Autodesk Fusion 360 part; units mm, degrees
sketch "Sketch1" plane through (0, 0, 0) normal (0, 0, 1) x (1, 0, 0)
  arc A0 (39.26, -24.3675) -> (42.26, -21.3675) centre (39.26, -21.3675) ccw
  circle A1 centre (38.26, -0.0995) radius 1.525
  circle A2 centre (-38.26, -20.3675) radius 1.75
  circle A3 centre (-38.26, 20.3675) radius 1.75
  line L0 (42.26, 21.3675) -> (42.26, -21.3675)
  arc A4 (-42.26, -21.3675) -> (-39.26, -24.3675) centre (-39.26, -21.3675) ccw
  line L1 (39.26, -24.3675) -> (-39.26, -24.3675)
  line L2 (-42.26, -21.3675) -> (-42.26, 21.3675)
  arc A5 (-39.26, 24.3675) -> (-42.26, 21.3675) centre (-39.26, 21.3675) ccw
  arc A6 (42.26, 21.3675) -> (39.26, 24.3675) centre (39.26, 21.3675) ccw
  circle A7 centre (38.26, 20.3675) radius 1.75
  circle A8 centre (-38.26, -0.0995) radius 1.525
  circle A9 centre (38.26, -20.3675) radius 1.75
  arc A10 (16.525, -9.1875) -> (15.025, -7.6875) centre (15.025, -9.1875) ccw
  arc A11 (-35.575, -12.1875) -> (-34.075, -13.6875) centre (-34.075, -12.1875) ccw
  line L3 (4.025, -7.6875) -> (15.025, -7.6875)
  arc A12 (-15.025, -7.6875) -> (-16.525, -9.1875) centre (-15.025, -9.1875) ccw
  line L4 (-16.525, -12.1875) -> (-16.525, -9.1875)
  line L5 (23.075, -13.6875) -> (34.075, -13.6875)
  line L6 (-15.025, -13.6875) -> (-4.025, -13.6875)
  arc A13 (21.575, -12.1875) -> (23.075, -13.6875) centre (23.075, -12.1875) ccw
  line L7 (-34.075, -7.6875) -> (-23.075, -7.6875)
  arc A14 (34.075, -13.6875) -> (35.575, -12.1875) centre (34.075, -12.1875) ccw
  line L8 (-34.075, -13.6875) -> (-23.075, -13.6875)
  line L9 (2.525, -12.1875) -> (2.525, -9.1875)
  arc A15 (35.575, -9.1875) -> (34.075, -7.6875) centre (34.075, -9.1875) ccw
  arc A16 (-2.525, -9.1875) -> (-4.025, -7.6875) centre (-4.025, -9.1875) ccw
  arc A17 (4.025, -7.6875) -> (2.525, -9.1875) centre (4.025, -9.1875) ccw
  line L10 (-35.575, -12.1875) -> (-35.575, -9.1875)
  line L11 (16.525, -12.1875) -> (16.525, -9.1875)
  arc A18 (-4.025, -13.6875) -> (-2.525, -12.1875) centre (-4.025, -12.1875) ccw
  line L12 (23.075, -7.6875) -> (34.075, -7.6875)
  arc A19 (-23.075, -13.6875) -> (-21.575, -12.1875) centre (-23.075, -12.1875) ccw
  line L13 (21.575, -12.1875) -> (21.575, -9.1875)
  line L14 (-15.025, -7.6875) -> (-4.025, -7.6875)
  line L15 (35.575, -12.1875) -> (35.575, -9.1875)
  arc A20 (2.525, -12.1875) -> (4.025, -13.6875) centre (4.025, -12.1875) ccw
  arc A21 (-16.525, -12.1875) -> (-15.025, -13.6875) centre (-15.025, -12.1875) ccw
  arc A22 (-21.575, -9.1875) -> (-23.075, -7.6875) centre (-23.075, -9.1875) ccw
  line L16 (-21.575, -12.1875) -> (-21.575, -9.1875)
  line L17 (-2.525, -12.1875) -> (-2.525, -9.1875)
  arc A23 (15.025, -13.6875) -> (16.525, -12.1875) centre (15.025, -12.1875) ccw
  arc A24 (-34.075, -7.6875) -> (-35.575, -9.1875) centre (-34.075, -9.1875) ccw
  line L18 (4.025, -13.6875) -> (15.025, -13.6875)
  arc A25 (23.075, -7.6875) -> (21.575, -9.1875) centre (23.075, -9.1875) ccw
  line L19 (-18.69, 4.8975) -> (-18.69, 13.8975)
  arc A26 (-18.69, 13.8975) -> (-21.69, 16.8975) centre (-21.69, 13.8975) ccw
  line L20 (-21.69, 16.8975) -> (-34.69, 16.8975)
  arc A27 (-34.69, 16.8975) -> (-37.69, 13.8975) centre (-34.69, 13.8975) ccw
  line L21 (-37.69, 4.8975) -> (-37.69, 13.8975)
  arc A28 (-37.69, 4.8975) -> (-34.69, 1.8975) centre (-34.69, 4.8975) ccw
  line L22 (-21.69, 1.8975) -> (-34.69, 1.8975)
  arc A29 (-21.69, 1.8975) -> (-18.69, 4.8975) centre (-21.69, 4.8975) ccw
  line L23 (35, -3.4325) -> (15, -3.4325)
  line L24 (19.67, 23.0675) -> (15, 23.0675)
  line L25 (30.33, 23.0675) -> (35, 23.0675)
  line L26 (15, -3.4325) -> (15, 23.0675)
  line L27 (35, 23.0675) -> (35, -3.4325)
  line L28 (19.67, 23.0675) -> (19.67, 24.3675)
  line L29 (30.33, 23.0675) -> (30.33, 24.3675)
  line L30 (39.26, 24.3675) -> (30.33, 24.3675)
  line L31 (19.67, 24.3675) -> (-39.26, 24.3675)
  point P0 (-42.26, -24.3675)
  dimension "d1" = 3.5
  dimension "d2" = 3.05
  dimension "d3" = 3.05
  dimension "d4" = 20.268
  dimension "d5" = 3
  dimension "d6" = 3
  dimension "d7" = 3
  dimension "d8" = 3
  dimension "d11" = 3.5
  dimension "d12" = 1.4142
  dimension "d13" = 4
  dimension "d14" = 10.68
  dimension "d15" = 6
  dimension "d16" = 14
  dimension "d17" = 1.5
  dimension "d18" = 1.5
  dimension "d19" = 1.5
  dimension "d20" = 1.5
  dimension "d21" = 1.5
  dimension "d22" = 1.5
  dimension "d23" = 1.5
  dimension "d24" = 1.5
  dimension "d25" = 1.5
  dimension "d26" = 1.5
  dimension "d27" = 1.5
  dimension "d28" = 1.5
  dimension "d29" = 1.5
  dimension "d30" = 1.5
  dimension "d31" = 1.5
  dimension "d32" = 1.5
  dimension "d33" = 6
  dimension "d34" = 6
  dimension "d35" = 6
  dimension "d36" = 10.68
  dimension "d37" = 10.68
  dimension "d38" = 10.68
  dimension "d40" = 6.685
  dimension "d41" = 5.05
  dimension "d42" = 5.05
  dimension "d43" = 5.05
  dimension "d44" = 4
  dimension "d45" = 4
  dimension "d46" = 4
  dimension "d47" = 1.4142
  dimension "d48" = 4
  dimension "d49" = 1.4142
  dimension "d50" = 20.268
  dimension "d51" = 14
  dimension "d52" = 14
  dimension "d53" = 14
  dimension "d54" = 6.685
  dimension "d55" = 3
  dimension "d56" = 3
  dimension "d57" = 3
  dimension "d58" = 3
  dimension "d59" = 19
  dimension "d60" = 15
  dimension "d61" = 4.57
  dimension "d63" = 26.5
  dimension "d64" = 26.5
  dimension "d65" = 20
  dimension "d66" = 10.66
  dimension "d67" = 1.3
  dimension "d68" = 1.3
  dimension "d69" = 4.67
  dimension "d70" = 4.67
  dimension "d71" = 7.26
  dimension "d78" = 3.5
  dimension "d79" = 3.5
extrude "Extrude1" add sketch "Sketch1" along normal blind 3
extrude "Extrude2" add 1 faces at (0.0405, 9.7541, 3) along direction (0, 0, 1) blind 4
extrude "Extrude4" add 1 faces at (0.0405, 9.7541, 7) along direction (0, 0, 1) blind 1
Geometry: final body of the model. Coordinates: model frame, mm. A direction names the side the tool comes from. Give positions to 0.01 mm unless a question says otherwise; leave off trailing zeros. Order: outer loops, then holes, each group sorted by start corner. A loop starts at its lowest first (then second) coordinate and runs counter-clockwise, first axis right, second up. Notation, with made-up numbers: (31, 11) - (58, 11) arc R33 cw to (58, 43) - close; hole circle Ø9 at (36, 46). An arc over 180 degrees is marked (long way). Use CSV: the item, a comma, the result in double quotes.
1. Section query C-C (x = -13.5). Output: boundary loops of the cut face in (y, z), plus the area to 3 significant figures.
Answers below:
outline,"(-24.37, 0) - (-13.69, 0) - (-13.69, 8) - (-24.37, 8) - close; (-7.69, 0) - (24.37, 0) - (24.37, 8) - (-7.69, 8) - close"
area,"342 mm2"
2. Access query for faces 4 (the face through (-28, 1.898, 4)), 5 (the face through (-42.26, 0, 4)). Directions: +Z, -Z, +X, -X, +Y, -Y. A direction counts if a zero-diameter tool reaches every point of the face in a straight line with its end or side. Return the directions, or none.
Answers below:
face 4,"+Z, -Z"
face 5,"+Z, -Z, -X, +Y, -Y"
3. Contact query for a flat-ended pin moving along its axis: pin 1 (1 mm diameter, centred on y = 23.5, z = 5, fed in from +X). Output: stop coordinate, or through.
Answers below:
pin 1,"x = 41.78"
4. Material intervals for line 1 along X through (y, z) = (-20.5, 3.25); line 2 along Y through (x, z) = (38.26, 6.25); line 3 along X through (y, z) = (13, 6.25), sorted ascending. Write a range as from..to.
Answers below:
line 1,"-42.26..-40, -36.52..36.52, 40..42.26"
line 2,"-24.37..-22.12, -18.62..-1.62, 1.43..18.62, 22.12..24.37"
line 3,"-42.26..-37.69, -18.69..15, 35..42.26"
5. Section query A-A (y = 8). Output: boundary loops of the cut face in (x, z), plus the area to 3 significant figures.
Answers below:
outline,"(-42.26, 0) - (-37.69, 0) - (-37.69, 8) - (-42.26, 8) - close; (-18.69, 0) - (15, 0) - (15, 8) - (-18.69, 8) - close; (35, 0) - (42.26, 0) - (42.26, 8) - (35, 8) - close"
area,"364 mm2"
6. Mould query, pull axis Y, two halves, no side actions, for faces 1 (the face through (42.26, 0, 4)), 2 (the face through (41.36, 23.51, 3.94)), 3 (the face through (33, 23.068, 4)). Classes: +Y half, -Y half, draft (parallel to the pull), parting line (faces both ways), or undercut.
Answers below:
face 1,"draft"
face 2,"+Y half"
face 3,"undercut"
7. Section query B-B (x = 38.26). Output: boundary loops of the cut face in (y, z), plus the area to 3 significant figures.
Answers below:
outline,"(-24.37, 0) - (-22.12, 0) - (-22.12, 8) - (-24.37, 8) - close; (-18.62, 0) - (-1.62, 0) - (-1.62, 8) - (-18.62, 8) - close; (1.43, 0) - (18.62, 0) - (18.62, 8) - (1.43, 8) - close; (22.12, 0) - (24.37, 0) - (24.37, 8) - (22.12, 8) - close"
area,"309 mm2"
8. Section query D-D (z = 2.75). Give the number of separate pieces and of enclosed holes in the cut face, plus the area to 3 significant figures.
Answers below:
separate pieces,"1"
enclosed holes,"11"
area,"2,910 mm2"
